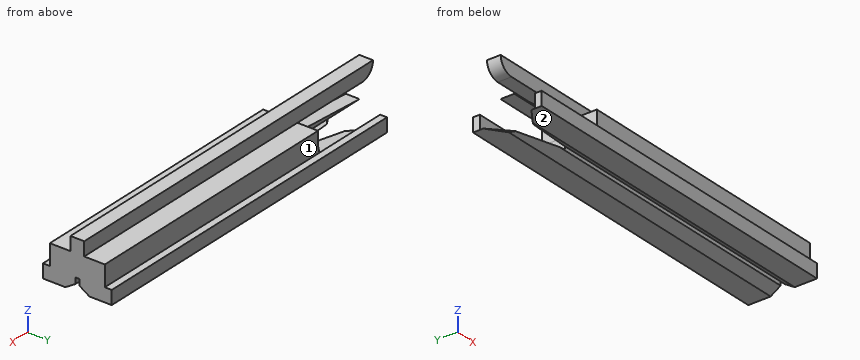
```python
from build123d import *

# Parameters (mm, degrees)
F0_W      = 30
F0_H      = 5
F1_DEPTH  = 8
F4_DEPTH  = 51.001
F5_DEPTH  = 5.001
F6_W      = 1
F6_H      = 2
F7_DEPTH  = 51
F8_W      = 2
F8_H      = 0.75
F9_DEPTH  = 11.5
F11_DEPTH = 6.001
F12_W     = 39.5
F12_H     = 2
F12_W_2   = 14
F13_DEPTH = 2
F14_R     = 1.99999


# Not quite as in the source:
# - a fillet or chamfer is up to 0.001 mm smaller than in the source, because OpenCascade refuses the exact size


with BuildPart() as f1:
    # F0 (on Front) → F1 (new body)
    with BuildSketch(Plane.XZ):
        Polygon((0, 0), (0, 5), (-9.5, 5), (-9.5, 3), (-10, 1), (-21, 0), align=None)
        with Locations((15, 2.5)):
            Rectangle(F0_W, F0_H)
    extrude(amount=F1_DEPTH)

    # F3 (on face) → F4 (cut, through all)
    with BuildSketch(Plane.YZ.offset(30)):
        Polygon((-3.7, 1.8), (-4.3, 1.8), (-4.3, 0.9114285714), (-4, 1.1), (-3.7, 0.9114285714), align=None)
        Polygon((-4.3, 0), (-4.3, 0.9114285714), (-5.75, 0), align=None)
        Polygon((-2.25, 0), (-3.7, 0.9114285714), (-3.7, 0), align=None)
        Polygon((-4, 1.1), (-4.3, 0.9114285714), (-4.3, 0), (-3.7, 0), (-3.7, 0.9114285714), align=None)
    extrude(amount=-F4_DEPTH, mode=Mode.SUBTRACT)

    # F2 (on face) → F5 (cut, through all)
    with BuildSketch(Plane(origin=(0, 0, 0), x_dir=(1, 0, 0), z_dir=(0, 0, -1))):
        Polygon((-16, 4), (-21, 7.5), (-21, 0.5), align=None)
    extrude(amount=-F5_DEPTH, mode=Mode.SUBTRACT)

    # F6 (on face) → F7 (join, through all)
    with BuildSketch(Plane.YZ.offset(30)):
        with Locations((-8.5, 1)):
            Rectangle(F6_W, F6_H)
        with Locations((0.5, 1)):
            Rectangle(F6_W, F6_H)
    extrude(amount=-F7_DEPTH)

    # F8 (on face) → F9 (join)
    with BuildSketch(Plane(origin=(-9.5, 0, 0), x_dir=(0, -1, 0), z_dir=(-1, 0, 0))):
        with Locations((4, 3.375)):
            Rectangle(F8_W, F8_H)
    extrude(amount=F9_DEPTH)

    # F10 (on face) → F11 (cut, through all)
    with BuildSketch(Plane.XZ.offset(5)):
        Polygon((-21, 3.75), (-21, 3), (-9.5, 3.75), align=None)
    extrude(amount=-F11_DEPTH, mode=Mode.SUBTRACT)

    # F12 (on face) → F13 (join)
    with BuildSketch(Plane.XY.offset(5)):
        with Locations((10.25, -4)):
            Rectangle(F12_W, F12_H)
        with Locations((-16.5, -4)):
            Rectangle(F12_W_2, F12_H)
    extrude(amount=F13_DEPTH)

    # F14 (radius 2 in the source; OpenCascade refuses exactly that, so slightly less here)
    f14_edges = [f1.edges().sort_by_distance(p)[0] for p in [
        (-23.5, -4, 5),
    ]]
    fillet(f14_edges, radius=F14_R)


solid = f1.part
```
Input: part model. Units: mm. Frame: model coordinates. Face numbers are marked on the shaded views. A direction names the side the tool comes from. Give positions to 0.01 mm unless a question says otherwise; leave off trailing zeros. Loops run counter-clockwise (first coordinate to the right, second up) from the corner with the lowest first, then second, coordinate; pieces in that order, holes last. Notation, with made-up numbers: M 28.5,5.5 L 42.5,5.5 A14 ccw 42.5,21.5 Z; hole C 18,60.25 d11. An arc over 180 degrees is marked long. Answer as CSV lines item,"result". Start each with the question number.
1. Section A-A on x = -5.5. Return loops of the section in (y, z).
2. Section D-D on z = 6.5. Return loops of the section in (x, y).
3. Reachability of the marked faces 1 and 2 from +Z, -Z, +X, -X, +Y, -Y: full face, straight path, thin tool, end or side. Return the list, or none.
4. Section B-B on x = -13.5. Return loops of the section in (y, z), plus the area to 3 significant figures.
5. Line query: L1, parallel to Y at x = -20.5, z = 0.5; L2, parallel to Y at x = 13, z = 1.5; L3, parallel to Z at x = 24, y = -1.5. Output: solid intervals per line, ascending.
6. Pin query (flat end, axial travel): P1, Ø4, axis at y = -5, z = 2, coming from the -X side; P2, Ø1, axis at y = -2.5, z = 2.5, coming from the -X side; P3, Ø0.6, axis at x = 15, z = 6.5, coming from the +Y side. Return the tip coordinate at first contact, or that it passes through.
7. Section C-C on z = 4.25. Return loops of the section in (x, y).
Computed values:
1,outline,"M -9,0 L -5.75,0 L -4.3,0.91 L -4.3,1.8 L -3.7,1.8 L -3.7,0.91 L -2.25,0 L 1,0 L 1,2 L 0,2 L 0,5 L -3,5 L -3,7 L -5,7 L -5,5 L -8,5 L -8,2 L -9,2 Z"
2,outline,"M -23.44,-5 L 30,-5 L 30,-3 L -23.44,-3 Z"
3,face 1,"+Z, +X, -X, +Y"
3,face 2,"-Z, +X, -X, +Y, -Y"
4,outline,"M -9,0 L -5.75,0 L -4.67,0.68 L -8,0.68 L -8,2 L -9,2 Z; M -5,3 L -3,3 L -3,3.49 L -5,3.49 Z; M -5,5 L -3,5 L -3,7 L -5,7 Z; M -3.33,0.68 L -2.25,0 L 1,0 L 1,2 L 0,2 L 0,0.68 Z"
4,area,"12.8 mm²"
5,L1,"y = -9 to -8, 0 to 1"
5,L2,"y = -9 to -4.3, -3.7 to 1"
5,L3,"z = 0 to 5"
6,P1,"stops at x = -21"
6,P2,"stops at x = -9.75"
6,P3,"stops at y = -3"
7,outline,"M -9.5,-8 L 30,-8 L 30,0 L -9.5,0 Z"
